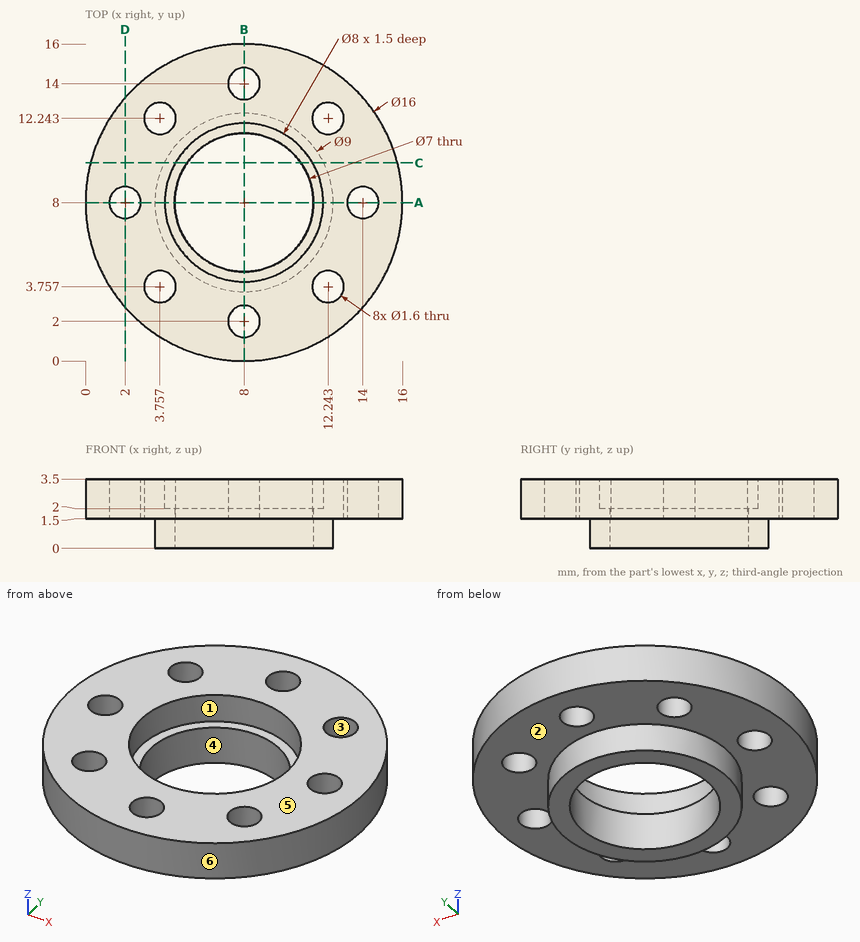
Could you check a few things on this drawing? It's one solid part, dimensions in mm from its lowest x, y, z. A direction names the side the tool comes from. Coordinates: 2 decimals unless noted, no trailing zeros. Write each loop counter-clockwise with the first axis right and the second up, starting at its lowest first coordinate (ties: lowest second). Pieces come first, ordered by that corner, then holes. Notation, with made-up numbers: (83.5, 61) - (113.5, 61) arc R21 cw to (113.5, 90) - close; hole circle Ø1 at (13.5, 16.25). An arc over 180 degrees is marked (long way). Write item = value, one per line.
1) Suppose I cut it at A-A on y = 8. Please give me the cut outline in (x, z).
Result set:
outline = (0, 1.5) - (1.2, 1.5) - (1.2, 3.5) - (0, 3.5) - close; (2.8, 1.5) - (3.5, 1.5) - (3.5, 0) - (4.5, 0) - (4.5, 2) - (4, 2) - (4, 3.5) - (2.8, 3.5) - close; (11.5, 0) - (12.5, 0) - (12.5, 1.5) - (13.2, 1.5) - (13.2, 3.5) - (12, 3.5) - (12, 2) - (11.5, 2) - close; (14.8, 1.5) - (16, 1.5) - (16, 3.5) - (14.8, 3.5) - close
2) Suppose I cut it at D-D on x = 2. Please give me the cut outline in (y, z).
Result set:
outline = (2.71, 1.5) - (7.2, 1.5) - (7.2, 3.5) - (2.71, 3.5) - close; (8.8, 1.5) - (13.29, 1.5) - (13.29, 3.5) - (8.8, 3.5) - close
3) For the marked faces 1, 2 and 3, which set-ups out of +Z, -Z, +X, -X, +Y, -Y let a thin tool reach every point of the face, with its end or its side?
Result set:
face_1 = +Z
face_2 = -Z
face_3 = +Z, -Z
4) Suppose I cut it at C-C on y = 10. Please give me the cut outline in (x, z), plus the area to 3 significant figures.
Result set:
outline = (0.25, 1.5) - (3.97, 1.5) - (3.97, 0) - (5.13, 0) - (5.13, 2) - (4.54, 2) - (4.54, 3.5) - (0.25, 3.5) - close; (10.87, 0) - (12.03, 0) - (12.03, 1.5) - (15.75, 1.5) - (15.75, 3.5) - (11.46, 3.5) - (11.46, 2) - (10.87, 2) - close
area = 21.2 mm2
5) Please list where these lines run through material, in increasing order: line 1 (Y direction, x = 8, z = 2.8); line 2 (Y direction, x = 3.25, z = 2.4) (1 decimal); line 3 (Z direction, x = 1.75, y = 6.25). Write a range as [from, to].
Result set:
line_1 = [0, 1.2], [2.8, 4], [12, 13.2], [14.8, 16]
line_2 = [1.6, 3.1], [4.4, 11.6], [12.9, 14.4]
line_3 = [1.5, 3.5]
6) Will these pins go through, and if not, where does the flat tip stop? pin 1 Ø6.5 at (x, y) = (8.5, 8.5) entering from +Z; pin 2 Ø1.4 at (x, y) = (12.24, 3.76) entering from +Z; pin 3 Ø2.5 at (x, y) = (8, 14) entering from -Z; pin 4 Ø2 at (x, y) = (12.24, 12.24) entering from +Z.
Result set:
pin_1 = 2
pin_2 = through
pin_3 = 1.5
pin_4 = 3.5
7) We'd pull the mould along Y, two halves only. Please class the marked faces 4, 5 and 6: +Y half, -Y half, draft (parallel to the pull), parting line (faces both ways), or undercut.
Result set:
face_4 = undercut
face_5 = draft
face_6 = parting line
